The listing builds one solid part. Answer for the finished solid, in the listing's coordinates (mm). Face numbers are marked on the shaded views. A direction names the side the tool comes from. Round coordinates to 2 decimals unless told otherwise and drop trailing zeros. Order: outer loops, then holes, each group sorted by start corner. A loop starts at its lowest first (then second) coordinate and runs counter-clockwise, first axis right, second up. Notation, with made-up numbers: (68, -19) -> (82, -19) arc R16 ccw to (82, 9) -> close; hole circle Ø2 at (83, 79). An arc over 180 degrees is marked (long way). Answer in a Markdown table with one row per item. Add a question column.
```python
from build123d import *

# Parameters (mm, degrees)
F0_W      = 88.9
F0_H      = 38.1
F1_DEPTH  = 50.8
F2_W      = 63.5
F2_H      = 25.4
F3_DEPTH  = 50.801
F5_DEPTH  = 25.4
F6_R      = 6.35
F8_DEPTH  = 12.701
F7_R      = 6.35
F9_DEPTH  = 25.401
F10_DEPTH = 38.102


with BuildPart() as f1:
    # F0 (on Front) → F1 (new body)
    with BuildSketch(Plane.XZ):
        with Locations((-5.6491568685, -3.2382767176)):
            Rectangle(F0_W, F0_H)
    extrude(amount=F1_DEPTH)

    # F2 (on face) → F3 (cut, through all)
    with BuildSketch(Plane.XZ.offset(50.8)):
        with Locations((-5.6491568685, 3.1117232824)):
            Rectangle(F2_W, F2_H)
    extrude(amount=-F3_DEPTH, mode=Mode.SUBTRACT)

    # F4 (on face) → F5 (cut)
    with BuildSketch(Plane.XZ.offset(50.8)):
        Polygon((26.1008431315, -9.5882767176), (0, -9.5882767176), (0, -22.2882767176), (38.8008431315, -22.2882767176), (38.8008431315, 15.8117232824), (26.1008431315, 15.8117232824), align=None)
    extrude(amount=-F5_DEPTH, mode=Mode.SUBTRACT)

    # F6 (on face) → F8 (cut, through all)
    with BuildSketch(Plane.XY.offset(-9.5882767176)):
        with Locations((0.7008431315, -12.7)):
            Circle(F6_R)
    extrude(amount=-F8_DEPTH, mode=Mode.SUBTRACT)

    # F7 (on face) → F9 (join, through all)
    with BuildSketch(Plane.XY.offset(-9.5882767176)):
        with Locations((-24.6991568685, -38.1)):
            Circle(F7_R)
    extrude(amount=F9_DEPTH)

    # F10 (cut, through all): a face of the model
    f10_faces = [f1.faces().sort_by_distance(p)[0] for p in [
        (-24.6991568685, -38.1, 15.8127232824),
    ]]
    extrude(f10_faces, amount=-F10_DEPTH, mode=Mode.SUBTRACT)


solid = f1.part
```
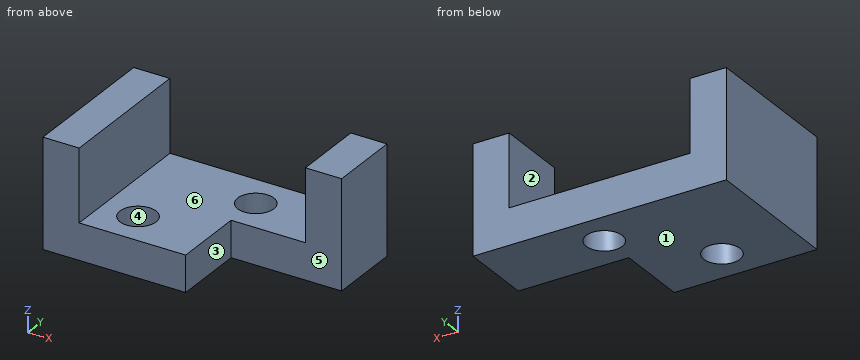
1. The mould has two halves that part along X. Classify the marked faces 1, 2 and 3: released by +X, released by -X, zero draft, split by the parting line, or undercut.
2. Each of these flat-tipped pins is pushed along its axis until it touches: pin 1 (19 mm diameter, centred on x = 27, z = -7.5, fed in from -Y); pin 2 (14.5 mm diameter, centred on x = 0.7, y = -12.7, fed in from +Z); pin 3 (10 mm diameter, centred on y = -35, z = -18, fed in from +X). Where does it stop, or does it pass through?
3. The part is cut by section D-D (x = 1.5). Give the vertices of the cut face in (y, z), then the cut area to 3 significant figures.
4. The part is cut by section B-B (y = -38.1). Give the vertices of the cut face in (x, z), then the cut area to 3 significant figures.
5. The part is cut by section A-A (z = 5.5). Give the vertices of the cut face in (x, y), then the cut area to 3 significant figures.
6. For the marked faces 4, 5 and 6, determine the directions among +Z, -Z, +X, -X, +Y, -Y from which every point of the face is accessible in a straight line to the end or side of a thin tool.
7. Straight lines are drawn through the part: line 1 along X through (y, z) = (-16, 14.5); line 2 along X through (y, z) = (-39.5, 2.5); line 3 along Y through (x, z) = (9.5, -13). For each, find the intervals that lie inside material, in ascending order.
8. The part is cut by section C-C (z = -16.5). Give the vertices of the cut face in (x, y).
Report:
| question | item | result |
|---|---|---|
| 1 | face 1 | zero draft |
| 1 | face 2 | undercut |
| 1 | face 3 | released by +X |
| 2 | pin 1 | stops at y = -25.4 |
| 2 | pin 2 | stops at z = -9.59 |
| 2 | pin 3 | stops at x = 0 |
| 3 | outline | (-25.4, -22.29) -> (-19, -22.29) -> (-19, -9.59) -> (-25.4, -9.59) -> close; (-6.4, -22.29) -> (0, -22.29) -> (0, -9.59) -> (-6.4, -9.59) -> close |
| 3 | area | 163 mm^2 |
| 4 | outline | (-50.1, -22.29) -> (-31.05, -22.29) -> (-31.05, -9.59) -> (-37.4, -9.59) -> (-37.4, 15.81) -> (-50.1, 15.81) -> close; (-18.35, -22.29) -> (0, -22.29) -> (0, -9.59) -> (-18.35, -9.59) -> close |
| 4 | area | 798 mm^2 |
| 5 | outline | (-50.1, -50.8) -> (-37.4, -50.8) -> (-37.4, 0) -> (-50.1, 0) -> close; (26.1, -25.4) -> (38.8, -25.4) -> (38.8, 0) -> (26.1, 0) -> close |
| 5 | area | 968 mm^2 |
| 6 | face 4 | +Z, -Z |
| 6 | face 5 | +Z, -Z, +X, -Y |
| 6 | face 6 | +Z, +Y, -Y |
| 7 | line 1 | x = -50.1 to -37.4, 26.1 to 38.8 |
| 7 | line 2 | x = -50.1 to -37.4 |
| 7 | line 3 | y = -25.4 to 0 |
| 8 | outline | (-50.1, -50.8) -> (0, -50.8) -> (0, -25.4) -> (38.8, -25.4) -> (38.8, 0) -> (-50.1, 0) -> close; hole circle Ø12.7 at (-24.7, -38.1); hole circle Ø12.7 at (0.7, -12.7) |
